Answer from the drawing. Dimensions are ordinates in mm from the lowest x, y and z of the part. A direction names the side the tool comes from. Coordinates: 2 decimals unless noted, no trailing zeros. Write each loop counter-clockwise with the first axis right and the second up, starting at its lowest first coordinate (ties: lowest second). Pieces come first, ordered by that corner, then holes. Notation, with made-up numbers: (36, 22.5) -> (89, 22.5) arc R30 ccw to (89, 54.5) -> close; hole circle Ø6 at (-29.5, -5). An arc over 180 degrees is marked (long way). Return JSON: item names as keys, results as strings.
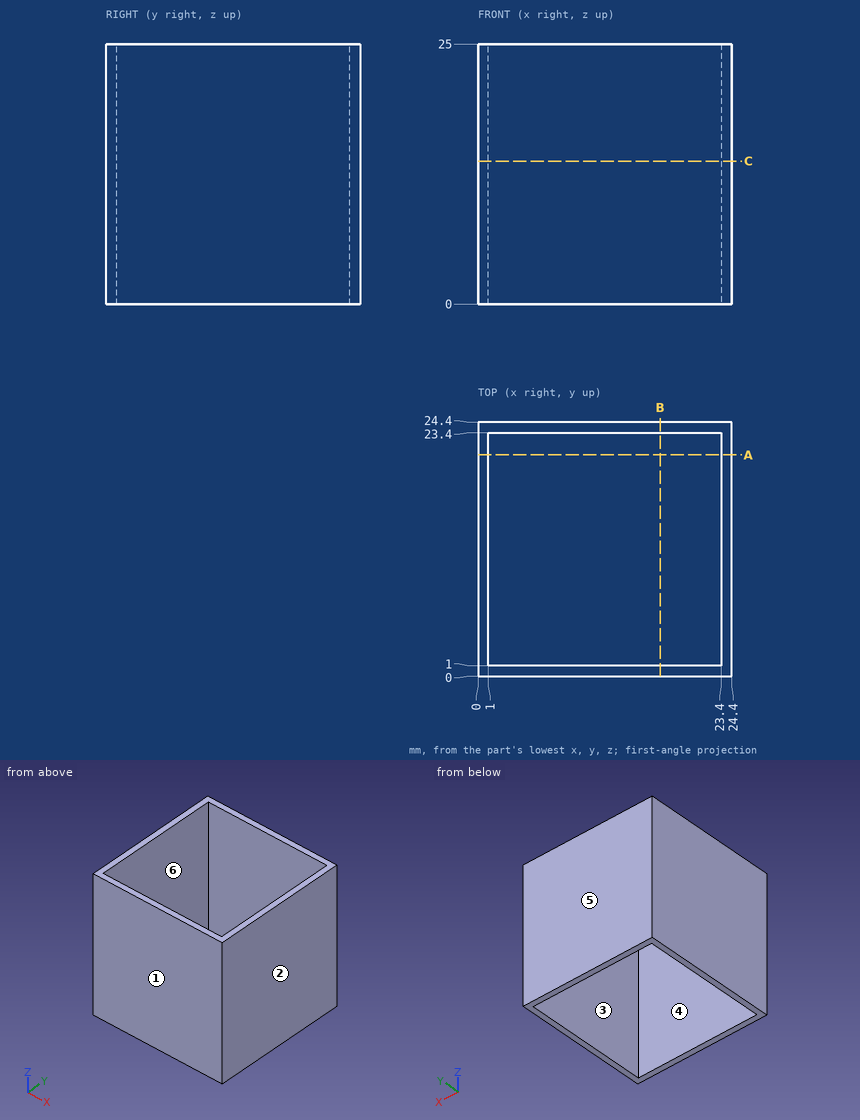
1. A tool of negligible diameter and unlimited length cuts with its end or side. For the marked faces 5 and 6, from which of +Z, -Z, +X, -X, +Y, -Y can it reach the whole face along a straight path? Write none if from no direction.
Taken from the geometry:
{"face 5": "+Z, -Z, +X, -X, +Y", "face 6": "+Z, -Z"}
2. For a pull along Y with two mould halves and no side action, classify the marked faces 1, 2, 3 and 4 as +Y half, -Y half, draft (parallel to the pull), parting line (faces both ways), or undercut.
Taken from the geometry:
{"face 1": "-Y half", "face 2": "draft", "face 3": "undercut", "face 4": "undercut"}
3. The part is cut by section C-C (z = 13.75). Determine the outline of the cut face in (x, y), then the cut area to 3 significant figures.
Taken from the geometry:
{"outline": "(0, 0) -> (24.4, 0) -> (24.4, 24.4) -> (0, 24.4) -> close; hole (1, 1) -> (23.4, 1) -> (23.4, 23.4) -> (1, 23.4) -> close", "area": "93.6 mm2"}
4. The part is cut by section A-A (y = 21.25). Determine the outline of the cut face in (x, z), then the cut area to 3 significant figures.
Taken from the geometry:
{"outline": "(0, 0) -> (1, 0) -> (1, 25) -> (0, 25) -> close; (23.4, 0) -> (24.4, 0) -> (24.4, 25) -> (23.4, 25) -> close", "area": "50.0 mm2"}
5. Consider L1, parallel to X at y = 15.5, z = 20. Determine where the line is inside the solid, lowest interval first.
Taken from the geometry:
{"L1": "x = 0 to 1, 23.4 to 24.4"}
